Read the model definition and answer for the solid it produces. Units are mm, in the model's axes. A direction names the side the tool comes from. Round coordinates to 2 decimals unless told otherwise and drop trailing zeros. Order: outer loops, then holes, each group sorted by start corner. A loop starts at its lowest first (then second) coordinate and runs counter-clockwise, first axis right, second up. Notation, with made-up numbers: (72, 9.25) -> (104, 9.25) arc R24 ccw to (104, 47.25) -> close; hole circle Ø8 at (12.25, 71). An arc over 180 degrees is marked (long way). Use a Markdown table: item, result. Add a question column.
1. Given pin 1 (1 mm diameter, centred on y = -3, z = 6, fed in from +X); pin 2 (0.8 mm diameter, centred on y = 0, z = 14, fed in from -X) (3 decimals); pin 3 (1.6 mm diameter, centred on x = 5.5, z = 17, fed in from -Y), each flat-ended and moving along its own axis, determine where each tip first touches the part or whether it passes through.
2. Section B-B, the plane y = 0 is taken. Give the vertices of the cut face in (x, z) (3 decimals), then the cut area to 3 significant figures.
3. Section A-A, the plane z = 6.75 is taken. Give the vertices of the cut face in (x, y) (3 decimals), then the cut area to 3 significant figures.
4. Section C-C, the plane x = 5 is taken. Give the vertices of the cut face in (y, z), then the cut area to 3 significant figures.
5. For faces 1 (the face through (-1.18, -2.09, 0.2)), 2 (the face through (-5, 0.913, 19)), 3 (the face through (-1.115, 1.896, 10.063)), 4 (the face through (5, 0.986, 18)), determine the directions among +Z, -Z, +X, -X, +Y, -Y from which every point of the face is accessible in a straight line to the end or side of a thin tool.
6. The mould has two halves that part along X. Classify faces 5 (the face through (1.18, 2.09, 0.2)), 6 (the face through (5, -1.014, 18)), 7 (the face through (4.04, -1.68, 10.37)): +X half, -X half, draft (parallel to the pull), parting line (faces both ways), or undercut.
7. Consider L1, parallel to X at y = 0, z = 11.5 (3 decimals); L2, parallel to Y at x = 0.25, z = 17.5; L3, parallel to X at y = -1.5, z = 17. Determine where each line is inside the solid, lowest interval first. Write a range as [from, to].
```python
from build123d import *

# Parameters (mm, degrees)
F0_R        = 4.375
F1_DEPTH    = 20
F2_W        = 2
F2_H        = 4
F3_DEPTH    = 3.5
F4_W        = 2
F4_H        = 4
F5_DEPTH    = 3.5
F6_T4_DEPTH = 16.4014247326
F6_S5_R     = 4.375
F6_T6_DEPTH = 10
F7_SIZE     = 1
F8_SIZE     = 0.4


# Not quite as in the source:
# - a fillet or chamfer that OpenCascade refuses, or shapes differently, is made with other operations: its cross-section is extruded or revolved along the edge and cut away or added


with BuildPart() as f1:
    # F0 (on Top) → F1 (new body)
    with BuildSketch(Plane.XY):
        Circle(F0_R)
        Polygon((-2.2, -1.2701705922), (-2.2, 1.2701705922), (0, 2.5403411844), (2.2, 1.2701705922), (2.2, -1.2701705922), (0, -2.5403411844), align=None, mode=Mode.SUBTRACT)
    extrude(amount=F1_DEPTH)

    # F2 (on face) → F3 (join)
    with BuildSketch(Plane.YZ.offset(-2.2)):
        with Locations((-0.0866705922, 18)):
            Rectangle(F2_W, F2_H)
    extrude(amount=-F3_DEPTH)

    # F4 (on face) → F5 (join)
    with BuildSketch(Plane(origin=(2.2, 0, 0), x_dir=(0, -1, 0), z_dir=(-1, 0, 0))):
        with Locations((0.0136538511, 18)):
            Rectangle(F4_W, F4_H)
    extrude(amount=-F5_DEPTH)

    # F6: chamfer of 2.8 on 1 edges, made by hand


with BuildPart() as f6_tool2:
    # F6_s3 → F6_t4 (new body)
    with BuildSketch(Plane.XZ.offset(8.2873829585)):
        Polygon((-5.7, 18.8), (-2.9, 16), (-5.7, 16), align=None)
    extrude(amount=-F6_T4_DEPTH)

    # F6_s5 → F6_t6 (cut, symmetric)
    with BuildSketch(Plane.XY.offset(17.4)):
        Circle(F6_S5_R)
    extrude(amount=F6_T6_DEPTH, both=True, mode=Mode.SUBTRACT)


with BuildPart() as f1_1:
    add(f1.part)

    # F6_t1: cut F6_tool2
    add(f6_tool2.part, mode=Mode.SUBTRACT)

    # F7
    f7_edges = [f1_1.edges().sort_by_distance(p)[0] for p in [
        (-4.375, 0, 0),
    ]]
    chamfer(f7_edges, length=F7_SIZE)

    # F8
    f8_edges = [f1_1.edges().sort_by_distance(p)[0] for p in [
        (2.2, 0, 0),
        (1.1, -1.905256, 0),
        (-1.1, -1.905256, 0),
        (-2.2, 0, 0),
        (-1.1, 1.905256, 0),
        (1.1, 1.905256, 0),
    ]]
    chamfer(f8_edges, length=F8_SIZE)


solid = f1_1.part
```
Verdict:
| question | item | result |
|---|---|---|
| 1 | pin 1 | stops at x = 3.59 |
| 1 | pin 2 | stops at x = -4.375 |
| 1 | pin 3 | stops at y = -1.01 |
| 2 | outline | (-5.7, 18.8) -> (-4.375, 17.475) -> (-4.375, 1) -> (-3.375, 0) -> (-2.6, 0) -> (-2.2, 0.4) -> (-2.2, 20) -> (-5.7, 20) -> close; (2.2, 0.4) -> (2.6, 0) -> (3.375, 0) -> (4.375, 1) -> (4.375, 16) -> (5.7, 16) -> (5.7, 20) -> (2.2, 20) -> close |
| 2 | area | 93.6 mm2 |
| 3 | outline | circle Ø8.75 at (0, 0); hole (-2.2, -1.27) -> (0, -2.54) -> (2.2, -1.27) -> (2.2, 1.27) -> (0, 2.54) -> (-2.2, 1.27) -> close |
| 3 | area | 43.4 mm2 |
| 4 | outline | (-1.01, 16) -> (0.99, 16) -> (0.99, 20) -> (-1.01, 20) -> close |
| 4 | area | 8.00 mm2 |
| 5 | face 1 | -Z |
| 5 | face 2 | +Z, -Z, -X, +Y |
| 5 | face 3 | +Z, -Z |
| 5 | face 4 | +Z, -Z, +X, +Y |
| 6 | face 5 | undercut |
| 6 | face 6 | draft |
| 6 | face 7 | parting line |
| 7 | L1 | x = [-4.375, -2.2], [2.2, 4.375] |
| 7 | L2 | y = [-4.37, -2.4], [2.4, 4.37] |
| 7 | L3 | x = [-4.11, -1.8], [1.8, 4.11] |
